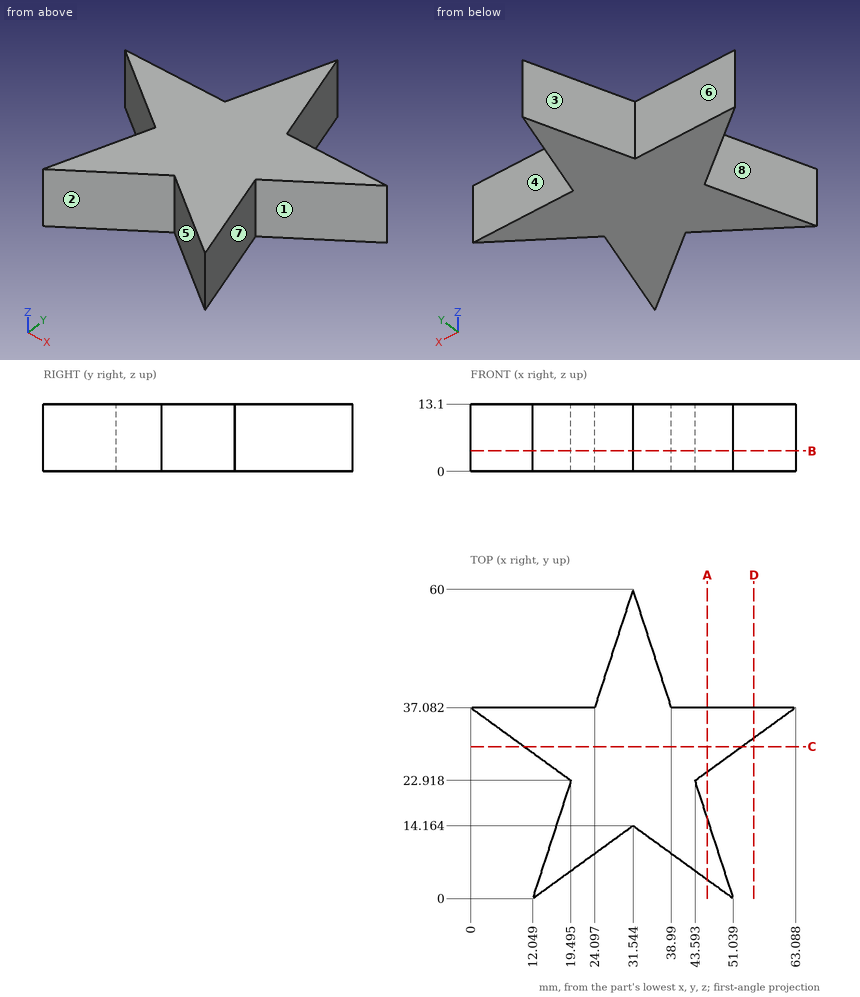
Job drawing, mm, ordinate dimensions from the low corner. One solid piece. A direction names the side the tool comes from. Give positions to 0.01 mm unless a question says otherwise; leave off trailing zeros. Loops run counter-clockwise (first coordinate to the right, second up) from the corner with the lowest first, then second, coordinate; pieces in that order, holes last. Notation, with made-up numbers: (74.5, 79.5) -> (109.5, 79.5) arc R27 cw to (109.5, 115.5) -> close; hole circle Ø7 at (60.25, -4). An arc over 180 degrees is marked (long way). Use a Markdown table: item, result. Add a question column.
(1) Wall check: line 1 along X through (y, z) = (10.5, 5.75) (1 decimal); line 2 along Y through (x, z) = (58.5, 5.5); line 3 along Y through (x, z) = (9, 7.5) (1 decimal). Give the ranges that are in metal, low to high.
(2) Slice it at C-C on y = 29.5. List the corners of the cut face in (x, z) (1 decimal), and give its area (3 significant figures).
(3) Drop flat-ended pins along their axis: pin 1 Ø4 at (x, z) = (7, 4) entering from +Y; pin 2 Ø6 at (x, y) = (42.5, 45) entering from -Z; pin 3 Ø1.5 at (y, z) = (23.5, 3.5) entering from +X (1 decimal); pin 4 Ø10 at (x, y) = (30, 14.5) entering from -Z. Give the stop position or say it passes through.
(4) Slice it at B-B on z = 4. List the corners of the cut face in (x, y) (1 decimal), and give its area (4 significant figures).
(5) Slice it at D-D on x = 55. List the corners of the cut face in (y, z).
(6) Tool access for the marked faces 4, 5, 6, 7 and 8: list every direction of +Z, -Z, +X, -X, +Y, -Y with a clear straight run to the whole face (end or side of a thin tool).
(7) Slice it at A-A on x = 46. List the corners of the cut face in (y, z), and give its area (3 significant figures).
(8) Mould opens along Y. For the marked faces 1, 2 and 3 say: +Y half, -Y half, draft (parallel to the pull), parting line (faces both ways), or undercut.
Filled sheet:
| question | item | result |
|---|---|---|
| 1 | line 1 | 15.5 to 26.5, 36.6 to 47.6 |
| 1 | line 2 | 33.75 to 37.08 |
| 1 | line 3 | 30.5 to 37.1 |
| 2 | outline | (10.4, 0) -> (52.7, 0) -> (52.7, 13.1) -> (10.4, 13.1) -> close |
| 2 | area | 553 mm2 |
| 3 | pin 1 | y = 37.08 |
| 3 | pin 2 | through |
| 3 | pin 3 | x = 45.4 |
| 3 | pin 4 | z = 0 |
| 4 | outline | (0, 37.1) -> (19.5, 22.9) -> (12, 0) -> (31.5, 14.2) -> (51, 0) -> (43.6, 22.9) -> (63.1, 37.1) -> (39, 37.1) -> (31.5, 60) -> (24.1, 37.1) -> close |
| 4 | area | 1,235 mm2 |
| 5 | outline | (31.21, 0) -> (37.08, 0) -> (37.08, 13.1) -> (31.21, 13.1) -> close |
| 6 | face 4 | +Z, -Z, +X, +Y |
| 6 | face 5 | +Z, -Z, -Y |
| 6 | face 6 | +Z, -Z, -X, +Y |
| 6 | face 7 | +Z, -Z, +X |
| 6 | face 8 | +Z, -Z, -X |
| 7 | outline | (3.66, 0) -> (15.51, 0) -> (15.51, 13.1) -> (3.66, 13.1) -> close; (24.67, 0) -> (37.08, 0) -> (37.08, 13.1) -> (24.67, 13.1) -> close |
| 7 | area | 318 mm2 |
| 8 | face 1 | undercut |
| 8 | face 2 | -Y half |
| 8 | face 3 | +Y half |
